Here's how the part is built. I have some questions about the finished solid (model axes, mm). A direction names the side the tool comes from. Give positions to 0.01 mm unless a question says otherwise; leave off trailing zeros. Write each loop counter-clockwise with the first axis right and the second up, starting at its lowest first coordinate (ties: lowest second). Pieces come first, ordered by that corner, then holes. Notation, with made-up numbers: (60, 17.5) -> (108, 17.5) arc R20 ccw to (108, 32.5) -> close; hole circle Ø4 at (-29.75, 40.25). An arc over 180 degrees is marked (long way). Answer as CSV lines item,"result". Start each with the question number.
from build123d import *

# Parameters (mm, degrees)
SKETCH1_R           = 11
BOSS_EXTRUDE1_DEPTH = 7
SKETCH2_W           = 5
SKETCH2_H           = 2.5
BOSS_EXTRUDE2_DEPTH = 13
CHAMFER2_SIZE       = 2
BOSS_EXTRUDE6_DEPTH = 2.5
CHAMFER3_SIZE       = 2
CHAMFER4_SIZE       = 2
BOSS_EXTRUDE4_DEPTH = 2.5
CHAMFER6_SIZE       = 2.5
CHAMFER7_SIZE       = 7
CHAMFER7_SIZE_2     = 13.165085257
CUT_EXTRUDE1_START  = -3
SKETCH6_R           = 1.5
CUT_EXTRUDE1_DEPTH  = 2.5
SKETCH7_R           = 1.5
CUT_EXTRUDE2_DEPTH  = 6


with BuildPart() as part:
    # Sketch1 → Boss-Extrude1 (new body)
    with BuildSketch(Plane.XY):
        Polygon((-15, 11.5), (-12.5, 14), (12.5, 14), (15, 11.5), (15, -14), (-15, -14), align=None)
        Circle(SKETCH1_R, mode=Mode.SUBTRACT)
    extrude(amount=BOSS_EXTRUDE1_DEPTH)

    # Sketch2 → Boss-Extrude2 (add)
    with BuildSketch(Plane(origin=(0, 0, 0), x_dir=(-1, 0, 0), z_dir=(0, 0, -1))):
        with Locations((-12.5, -12.75)):
            Rectangle(SKETCH2_W, SKETCH2_H)
        with Locations((12.5, -12.75)):
            Rectangle(SKETCH2_W, SKETCH2_H)
    extrude(amount=BOSS_EXTRUDE2_DEPTH)

    # Chamfer2
    chamfer2_edges = [part.edges().sort_by_distance(p)[0] for p in [
        (-10, -12.75, 0),
        (10, -12.75, 0),
    ]]
    chamfer(chamfer2_edges, length=CHAMFER2_SIZE)

    # Sketch5 → Boss-Extrude6 (add)
    with BuildSketch(Plane.XZ.offset(14)):
        Polygon((-10, -2), (-10, -7.5), (10, -7.5), (10, -2), (8, 0), (-8, 0), align=None)
    extrude(amount=-BOSS_EXTRUDE6_DEPTH)

    # Chamfer3
    chamfer3_edges = [part.edges().sort_by_distance(p)[0] for p in [
        (15, -1.25, 7),
    ]]
    chamfer(chamfer3_edges, length=CHAMFER3_SIZE)

    # Chamfer4
    chamfer4_edges = [part.edges().sort_by_distance(p)[0] for p in [
        (-15, -1.25, 7),
    ]]
    chamfer(chamfer4_edges, length=CHAMFER4_SIZE)

    # Sketch4 → Boss-Extrude4 (add)
    with BuildSketch(Plane(origin=(0, 0, 0), x_dir=(-1, 0, 0), z_dir=(0, 0, -1))):
        Polygon((-15, -1.25), (15, 11.5), (12.5, 14), (-12.5, 14), (-15, 11.5), align=None)
    extrude(amount=BOSS_EXTRUDE4_DEPTH)

    # Chamfer6
    # the kernel refuses this chamfer: 2.5 mm, written as the material it adds along each edge
    with BuildSketch(Plane(origin=(20.916998416, -3.764724327, 0), x_dir=(-0.39099275668343275, -0.9199829569021947, 0.02749587661058635), z_dir=(-0.9203309184584746, 0.39114064034485174, 0))) as chamfer6_piece_1_section:
        Polygon((CHAMFER6_SIZE * 0.999621916911, -CHAMFER6_SIZE * 0.0274958766106), (-CHAMFER6_SIZE * 0.0274958766106, -CHAMFER6_SIZE * 0.999621916911), (0, 0), align=None)
    chamfer6_piece_1 = extrude(amount=17.214861222, mode=Mode.PRIVATE)
    chamfer6_piece_1 = chamfer6_piece_1 - Plane(origin=(0, 0, -0.830769879), x_dir=(1, 0, 0), z_dir=(0, 0, -1)) * Cylinder(11, 45, mode=Mode.PRIVATE)
    chamfer6_piece_1 = split(chamfer6_piece_1, bisect_by=Plane(origin=(15, -1.305255327, -0.830769879), z_dir=(-1, 0, 0)), keep=Keep.TOP, mode=Mode.PRIVATE)
    add(chamfer6_piece_1)
    with BuildSketch(Plane(origin=(-1.383846422, 5.71313473, 0), x_dir=(-0.39099275668343275, -0.9199829569021946, 0.02749587661058637), z_dir=(-0.9203309184584746, 0.39114064034485174, 0))) as chamfer6_piece_2_section:
        Polygon((CHAMFER6_SIZE * 0.999621916911, -CHAMFER6_SIZE * 0.0274958766106), (-CHAMFER6_SIZE * 0.0274958766106, -CHAMFER6_SIZE * 0.999621916911), (0, 0), align=None)
    chamfer6_piece_2 = extrude(amount=21.224052785, mode=Mode.PRIVATE)
    chamfer6_piece_2 = chamfer6_piece_2 - Plane(origin=(0, 0, -0.851096237), x_dir=(1, 0, 0), z_dir=(0, 0, -1)) * Cylinder(11, 53, mode=Mode.PRIVATE)
    chamfer6_piece_2 = split(chamfer6_piece_2, bisect_by=Plane(origin=(-15, 9.126408424, -0.851096237), z_dir=(1, 0, 0)), keep=Keep.TOP, mode=Mode.PRIVATE)
    add(chamfer6_piece_2)

    # Chamfer7
    # the kernel refuses this chamfer: 13.165085257, 7 mm, written as the material it adds along each edge
    with BuildSketch(Plane(origin=(-15, -11.5, 0), x_dir=(0, 0.9979482451756082, 0.06402577567608186), z_dir=(1, 0, 0))) as chamfer7_piece_1_section:
        Polygon((CHAMFER7_SIZE * 0.997948245176, -CHAMFER7_SIZE * 0.0640257756761), (-CHAMFER7_SIZE_2 * 0.0640257756781, -CHAMFER7_SIZE_2 * 0.997948245208), (0, 0), align=None)
    chamfer7_piece_1 = extrude(amount=30, mode=Mode.PRIVATE)
    chamfer7_piece_1 = chamfer7_piece_1 - Plane(origin=(0, 0, -3.073682767), x_dir=(1, 0, 0), z_dir=(0, 0, -1)) * Cylinder(11, 113, mode=Mode.PRIVATE)
    chamfer7_piece_1 = split(chamfer7_piece_1, bisect_by=Plane(origin=(-12.500128058, -8.887755394, -7.5), z_dir=(0, 0, 1)), keep=Keep.TOP, mode=Mode.PRIVATE)
    chamfer7_piece_1 = split(chamfer7_piece_1, bisect_by=Plane(origin=(-10, -8.887755394, -3.073682767), z_dir=(-1, 0, 0)), keep=Keep.TOP, mode=Mode.PRIVATE)
    add(chamfer7_piece_1)
    with BuildSketch(Plane(origin=(-15, -11.5, 0), x_dir=(0, 0.9979482451756082, 0.06402577567608186), z_dir=(1, 0, 0))) as chamfer7_piece_2_section:
        Polygon((CHAMFER7_SIZE * 0.997948245176, -CHAMFER7_SIZE * 0.0640257756761), (-CHAMFER7_SIZE_2 * 0.0640257756781, -CHAMFER7_SIZE_2 * 0.997948245208), (0, 0), align=None)
    chamfer7_piece_2 = extrude(amount=30, mode=Mode.PRIVATE)
    chamfer7_piece_2 = split(chamfer7_piece_2, bisect_by=Plane(origin=(-12.5, -10.721530873, -7.5), z_dir=(0, 0, -1)), keep=Keep.TOP, mode=Mode.PRIVATE)
    chamfer7_piece_2 = split(chamfer7_piece_2, bisect_by=Plane(origin=(-10, -10.721530873, -9.597564575), z_dir=(-1, 0, 0)), keep=Keep.TOP, mode=Mode.PRIVATE)
    chamfer7_piece_2 = split(chamfer7_piece_2, bisect_by=Plane(origin=(-12.5, -10.721530873, -13), z_dir=(0, 0, 1)), keep=Keep.TOP, mode=Mode.PRIVATE)
    add(chamfer7_piece_2)
    with BuildSketch(Plane(origin=(-15, -11.5, 0), x_dir=(0, 0.9979482451756082, 0.06402577567608186), z_dir=(1, 0, 0))) as chamfer7_piece_3_section:
        Polygon((CHAMFER7_SIZE * 0.997948245176, -CHAMFER7_SIZE * 0.0640257756761), (-CHAMFER7_SIZE_2 * 0.0640257756781, -CHAMFER7_SIZE_2 * 0.997948245208), (0, 0), align=None)
    chamfer7_piece_3 = extrude(amount=30, mode=Mode.PRIVATE)
    chamfer7_piece_3 = chamfer7_piece_3 - Plane(origin=(0, 0, -3.793876077), x_dir=(1, 0, 0), z_dir=(0, 0, -1)) * Cylinder(11, 113, mode=Mode.PRIVATE)
    chamfer7_piece_3 = split(chamfer7_piece_3, bisect_by=Plane(origin=(-9.499486782, -6.598719884, -7.5), z_dir=(0, 0, 1)), keep=Keep.TOP, mode=Mode.PRIVATE)
    chamfer7_piece_3 = split(chamfer7_piece_3, bisect_by=Plane(origin=(10, -6.598719884, -3.793876077), z_dir=(-1, 0, 0)), keep=Keep.TOP, mode=Mode.PRIVATE)
    chamfer7_piece_3 = split(chamfer7_piece_3, bisect_by=Plane(origin=(-10, -6.598719884, -3.793876077), z_dir=(1, 0, 0)), keep=Keep.TOP, mode=Mode.PRIVATE)
    add(chamfer7_piece_3)
    with BuildSketch(Plane(origin=(-15, -11.5, 0), x_dir=(0, 0.9979482451756082, 0.06402577567608186), z_dir=(1, 0, 0))) as chamfer7_piece_4_section:
        Polygon((CHAMFER7_SIZE * 0.997948245176, -CHAMFER7_SIZE * 0.0640257756761), (-CHAMFER7_SIZE_2 * 0.0640257756781, -CHAMFER7_SIZE_2 * 0.997948245208), (0, 0), align=None)
    chamfer7_piece_4 = extrude(amount=30, mode=Mode.PRIVATE)
    chamfer7_piece_4 = split(chamfer7_piece_4, bisect_by=Plane(origin=(12.5, -10.721530873, -7.5), z_dir=(0, 0, -1)), keep=Keep.TOP, mode=Mode.PRIVATE)
    chamfer7_piece_4 = split(chamfer7_piece_4, bisect_by=Plane(origin=(10, -10.721530873, -9.597564575), z_dir=(1, 0, 0)), keep=Keep.TOP, mode=Mode.PRIVATE)
    chamfer7_piece_4 = split(chamfer7_piece_4, bisect_by=Plane(origin=(12.5, -10.721530873, -13), z_dir=(0, 0, 1)), keep=Keep.TOP, mode=Mode.PRIVATE)
    add(chamfer7_piece_4)
    with BuildSketch(Plane(origin=(-15, -11.5, 0), x_dir=(0, 0.9979482451756082, 0.06402577567608186), z_dir=(1, 0, 0))) as chamfer7_piece_5_section:
        Polygon((CHAMFER7_SIZE * 0.997948245176, -CHAMFER7_SIZE * 0.0640257756761), (-CHAMFER7_SIZE_2 * 0.0640257756781, -CHAMFER7_SIZE_2 * 0.997948245208), (0, 0), align=None)
    chamfer7_piece_5 = extrude(amount=30, mode=Mode.PRIVATE)
    chamfer7_piece_5 = chamfer7_piece_5 - Plane(origin=(0, 0, -3.073682766), x_dir=(1, 0, 0), z_dir=(0, 0, -1)) * Cylinder(11, 113, mode=Mode.PRIVATE)
    chamfer7_piece_5 = split(chamfer7_piece_5, bisect_by=Plane(origin=(12.500128057, -8.887755394, -7.5), z_dir=(0, 0, 1)), keep=Keep.TOP, mode=Mode.PRIVATE)
    chamfer7_piece_5 = split(chamfer7_piece_5, bisect_by=Plane(origin=(10, -8.887755394, -3.073682766), z_dir=(1, 0, 0)), keep=Keep.TOP, mode=Mode.PRIVATE)
    add(chamfer7_piece_5)

    # Sketch6 → Cut-Extrude1 (cut)
    # profile 1 of 2: a face of its own
    with BuildSketch(Plane.XZ.offset(14).offset(CUT_EXTRUDE1_START)):
        Polygon((-8.3, 0.941154273), (-8.3, 4.058845727), (-11, 5.617691454), (-13.7, 4.058845727), (-13.7, 0.941154273), (-11, -0.617691454), align=None)
        with Locations(Location((-11, 2.5, 0), (0, 0, 270))):
            Circle(SKETCH6_R, mode=Mode.SUBTRACT)
    # profile 2 of 2: a face of its own
    with BuildSketch(Plane.XZ.offset(14).offset(CUT_EXTRUDE1_START)):
        Polygon((11, -0.617691454), (8.3, 0.941154273), (8.3, 4.058845727), (11, 5.617691454), (13.7, 4.058845727), (13.7, 0.941154273), align=None)
    extrude(amount=-CUT_EXTRUDE1_DEPTH, mode=Mode.SUBTRACT)

    # Sketch7 → Cut-Extrude2 (cut)
    with BuildSketch(Plane.XZ.offset(14)):
        with Locations(Location((11, 2.5, 0), (0, 0, 270))):
            Circle(SKETCH7_R)
        with Locations(Location((-11, 2.5, 0), (0, 0, 270))):
            Circle(SKETCH7_R)
    extrude(amount=-CUT_EXTRUDE2_DEPTH, mode=Mode.SUBTRACT)


solid = part.part
Item 1: For faces 4 (the face through (-12.33, -8.25, 1.81)), 5 (the face through (-11.59, 8.67, -1.23)), 6 (the face through (-2.017, -10.813, 1.26)), 7 (the face through (-10, -12, -10)), 8 (the face through (12.33, -9.77, 4.85)), which set-ups out of +Z, -Z, +X, -X, +Y, -Y let a thin tool reach every point of the face, with its end or its side?
Item 2: We'd pull the mould along Y, two halves only. Please class faces 1 (the face through (14, 0, 6)), 2 (the face through (12, -8.5, 4)), 3 (the face through (0, -14, -1)): released by +Y, released by -Y, zero draft, split by the parting line, or undercut.
Item 3: If we section it at B-B (x = 0.5): Please give me the cut outline in (y, z), and give its area (3 significant figures).
Item 4: I'm going to push flat-ended pins straight in: pin 1 (8 mm diameter, centred on y = -3.5, z = -2.5, fed in from -X); pin 2 (1.5 mm diameter, centred on x = -11.5, z = 3, fed in from -Y); pin 3 (2.5 mm diameter, centred on x = 11.5, y = -3.5, fed in from -Z); pin 4 (5 mm diameter, centred on x = -11.5, y = 1.5, fed in from -Z). Where does each tip first touch, or does it pass through?
Item 5: If we section it at A-A (y = -9.75): Please give me the cut outline in (x, z).
Item 6: If I drill on line 1 (X direction, y = -12.1, z = 2.5); line 2 (X direction, y = -8.75, z = 1.75); line 3 (X direction, y = -8.15, z = 2.5), over which ranges is the centre line in solid material (lowest first)? Write a range as [from, to].
Item 7: If we section it at C-C (z = -11): Please give me the cut outline in (x, y).
Final values:
1,face 4,"-Y"
1,face 5,"-Z, -X"
1,face 6,"+Z"
1,face 7,"-Z, +Y, -Y"
1,face 8,"none"
2,face 1,"zero draft"
2,face 2,"undercut"
2,face 3,"released by -Y"
3,outline,"(-14, -7.5) -> (-10.99, -7.5) -> (-10.99, 7) -> (-14, 7) -> close; (4.91, -2.5) -> (14, -2.5) -> (14, 7) -> (10.99, 7) -> (10.99, 0) -> (4.91, 0) -> close"
3,area,"87.5 mm2"
4,pin 1,"x = -15"
4,pin 2,"y = -8"
4,pin 3,"z = -0.47"
4,pin 4,"z = 0"
5,outline,"(-15, -9.87) -> (-10, -9.87) -> (-10, -7.5) -> (-5.09, -7.5) -> (-5.09, 7) -> (-13, 7) -> (-15, 5) -> close; (5.09, -7.5) -> (10, -7.5) -> (10, -9.87) -> (15, -9.87) -> (15, 5) -> (13, 7) -> (5.09, 7) -> close; hole (-13.7, 0.94) -> (-11, -0.62) -> (-8.3, 0.94) -> (-8.3, 4.06) -> (-11, 5.62) -> (-13.7, 4.06) -> close; hole (8.3, 0.94) -> (11, -0.62) -> (13.7, 0.94) -> (13.7, 4.06) -> (11, 5.62) -> (8.3, 4.06) -> close"
6,line 1,"[-15, -12.5], [-9.5, 9.5], [12.5, 15]"
6,line 2,"[-15, -13.7], [-8.3, -6.67], [6.67, 8.3], [13.7, 15]"
6,line 3,"[-15, -12.5], [-9.5, -7.39], [7.39, 9.5], [12.5, 15]"
7,outline,"(-15, -14) -> (-10, -14) -> (-10, -10.35) -> (-15, -10.35) -> close; (10, -14) -> (15, -14) -> (15, -10.35) -> (10, -10.35) -> close"
